Autodesk Inventor part; units mm, degrees
ref_plane "YZ Plane" through (0, 0, 0) normal (1, 0, 0) x (0, 1, 0)
ref_plane "XZ Plane" through (0, 0, 0) normal (0, 1, 0) x (-1, 0, 0)
ref_plane "XY Plane" through (0, 0, 0) normal (0, 0, 1) x (1, 0, 0)
sketch "Sketch1" plane through (0, 0, 0) normal (0, 1, 0) x (-1, 0, 0)
  line L0 (0, 0) -> (233.045, 0)
  line L1 (233.045, 0) -> (233.045, -38.1)
  line L2 (233.045, -38.1) -> (0, -38.1)
  line L3 (0, -38.1) -> (0, 0)
  dimension "d0" = 233.045
  dimension "d1" = 38.1
extrude "Extrusion1" add sketch "Sketch1" along normal blind 3.2766
sketch "Sketch2" plane through (0, 3.2766, 0) normal (0, 1, 0) x (1, 0, 0)
  line L0 (-7.62, 7.62) -> (-210.82, 7.62)
  line L1 (-210.82, 7.62) -> (-210.82, 30.48)
  line L2 (-210.82, 30.48) -> (-7.62, 30.48)
  line L3 (-7.62, 30.48) -> (-7.62, 7.62)
  point P0 (0, 0)
  dimension "d4" = 203.2
  dimension "d5" = 22.86
extrude "Extrusion2" cut sketch "Sketch2" against normal through all
fillet "Face Fillet1" radius 7.62 1 edges at (-210.82, 1.6383, -30.48)
fillet "Face Fillet2" radius 7.62 1 edges at (-210.82, 1.6383, -7.62)
fillet "Face Fillet3" radius 7.62 1 edges at (-7.62, 1.6383, -30.48)
fillet "Face Fillet4" radius 7.62 1 edges at (-7.62, 1.6383, -7.62)
sketch "Sketch3" plane through (-233.045, 0, 0) normal (0, 0, 1) x (1, 0, 0)
  line L0 (233.045, -4.826) -> (233.045, 7.8895)
  line L1 (233.045, 7.8895) -> (236.9365, 4.6242)
  line L2 (233.045, -4.826) -> (236.9365, -1.5606)
  line L3 (233.045, -4.826) -> (238.125, -4.826) construction
  line L4 (236.9365, -1.5606) -> (236.9365, 4.6242)
  line L5 (0, 7.8895) -> (0, -4.826)
  line L6 (0, -4.826) -> (-3.8915, -1.5606)
  line L7 (0, 7.8895) -> (-3.8915, 4.6242)
  line L8 (-3.8915, -1.5606) -> (-3.8915, 4.6242)
  point P0 (233.045, 0)
  dimension "d12" = 5.08
  dimension "d13" = 50
  dimension "d14" = 5.08
  dimension "d15" = 40
  dimension "d16" = 5.08
  dimension "d17" = 50
  dimension "d18" = 5.08
extrude "Extrusion3" add sketch "Sketch3" against normal blind 38.1
properties part number "short slider"
Design review of the part built by this model. Coordinates are the model's own, in mm. A direction names the side the tool comes from. Give positions to 0.01 mm unless a question says otherwise; leave off trailing zeros. Write each loop counter-clockwise with the first axis right and the second up, starting at its lowest first coordinate (ties: lowest second). Pieces come first, ordered by that corner, then holes.
(1) Clearance check with flat-ended pins moving along their axes: pin 1 Ø2.5 at (y, z) = (5.5, -28.5) entering from -X; pin 2 Ø2.5 at (y, z) = (-3, -26.5) entering from +X; pin 3 Ø2 at (x, y) = (-33.5, -2.5) entering from +Z; pin 4 Ø8 at (x, z) = (-212, -26) entering from +Y. State where each tip first meets the part, or that it passes through.
Checked values:
pin 1: stops at x = -236.94
pin 2: stops at x = 3.67
pin 3: passes through
pin 4: stops at y = 3.28
(2) Add section D-D (x = -87). Give the boundary of the cut face in (y, z).
Checked values:
outline: (0, -38.1) - (3.28, -38.1) - (3.28, -30.48) - (0, -30.48) - close; (0, -7.62) - (3.28, -7.62) - (3.28, 0) - (0, 0) - close
(3) Add section B-B (x = -207). Give the boundary of the cut face in (y, z).
Checked values:
outline: (0, -38.1) - (3.28, -38.1) - (3.28, -29.46) - (0, -29.46) - close; (0, -8.64) - (3.28, -8.64) - (3.28, 0) - (0, 0) - close
(4) Add section A-A (z = -20). Give the boundary of the cut face in (x, y) (1 decimal).
Checked values:
outline: (-236.9, -1.6) - (-233, -4.8) - (-233, 0) - (-210.8, 0) - (-210.8, 3.3) - (-233, 3.3) - (-233, 7.9) - (-236.9, 4.6) - close; (-7.6, 0) - (0, 0) - (0, -4.8) - (3.9, -1.6) - (3.9, 4.6) - (0, 7.9) - (0, 3.3) - (-7.6, 3.3) - close
(5) Wall thickness on line 1 along X through (y, z) = (-1.5, -32.5) (1 decimal); line 2 along Z through (x, y) = (-172.5, 1.5); line 3 along Y through (x, z) = (-9, -3.5): over which ranges is each line inside the solid? List them lowest first.
Checked values:
line 1: x = -236.9 to -233, 0 to 3.9
line 2: z = -38.1 to -30.48, -7.62 to 0
line 3: y = 0 to 3.28
(6) Tool access review of faces 4 (the face through (-117, 2, 0)), 5 (the face through (-236.936, 1, -19)), 6 (the face through (-208.647, 1.615, -28.189)), 7 (the face through (0, -2, -19)), 8 (the face through (0, 6, -19)): name each direction out of +Z, -Z, +X, -X, +Y, -Y from which nothing blocks a thin tool from reaching the whole face with its end or side.
Checked values:
face 4: +Z, +X, -X, +Y, -Y
face 5: +Z, -Z, -X, +Y, -Y
face 6: +Y, -Y
face 7: +Z, -Z, -Y
face 8: +Z, -Z, +Y
(7) Add section C-C (z = -4.5). Give the boundary of the cut face in (x, y) (1 decimal).
Checked values:
outline: (-236.9, -1.6) - (-233, -4.8) - (-233, 0) - (0, 0) - (0, -4.8) - (3.9, -1.6) - (3.9, 4.6) - (0, 7.9) - (0, 3.3) - (-233, 3.3) - (-233, 7.9) - (-236.9, 4.6) - close
(8) Mouldability with a two-part tool opening along Z and no side actions: class faces 1 (the face through (3.892, 1, -19)), 2 (the face through (-208.529, 1.615, -9.793)), 3 (the face through (-117, 2, -38.1)) as +Z half, -Z half, draft (parallel to the pull), parting line (faces both ways), or undercut.
Checked values:
face 1: draft
face 2: undercut
face 3: -Z half
